Check sheet for the modelled part. Datum: model origin and axes. Units: mm. A direction names the side the tool comes from. Round coordinates to 2 decimals unless told otherwise and drop trailing zeros. Loops run counter-clockwise (first coordinate to the right, second up) from the corner with the lowest first, then second, coordinate; pieces in that order, holes last. Notation, with made-up numbers: (75, -37) - (86, -37) arc R21 cw to (86, -33) - close; hole circle Ø2 at (-14.75, 66). An arc over 180 degrees is marked (long way). Put each result on its own line as item: value.
```python
from build123d import *

# Parameters (mm, degrees)
SKETCH1_W           = 10
SKETCH1_H           = 32
BOSS_EXTRUDE1_DEPTH = 4
SKETCH2_R           = 2.5
CUT_EXTRUDE1_DEPTH  = 4
SKETCH3_W           = 10
SKETCH3_H           = 3
BOSS_EXTRUDE2_DEPTH = 28.76
SKETCH4_W           = 2.542985542
SKETCH4_H           = 9.222544282
BOSS_EXTRUDE3_DEPTH = 3
SKETCH5_R           = 2
CUT_EXTRUDE2_DEPTH  = 13


with BuildPart() as part:
    # Sketch1 → Boss-Extrude1 (new body)
    with BuildSketch(Plane(origin=(0, 0, 0), x_dir=(1, 0, 0), z_dir=(0, 1, 0))):
        with Locations((5, 16)):
            Rectangle(SKETCH1_W, SKETCH1_H)
    extrude(amount=BOSS_EXTRUDE1_DEPTH)

    # Sketch2 → Cut-Extrude1 (cut)
    with BuildSketch(Plane(origin=(0, 4, 0), x_dir=(1, 0, 0), z_dir=(0, 1, 0))):
        with Locations((5, 10)):
            Circle(SKETCH2_R)
    extrude(amount=-CUT_EXTRUDE1_DEPTH, mode=Mode.SUBTRACT)

    # Sketch3 → Boss-Extrude2 (add)
    with BuildSketch(Plane(origin=(0, 4, 0), x_dir=(1, 0, 0), z_dir=(0, 1, 0))):
        with Locations((5, 30.5)):
            Rectangle(SKETCH3_W, SKETCH3_H)
    extrude(amount=BOSS_EXTRUDE2_DEPTH)

    # Sketch4 → Boss-Extrude3 (add)
    with BuildSketch(Plane.XY.offset(-29)):
        Polygon((10, 37.329817811), (10, 46.552362093), (0, 46.552362093), (0, 29.76), (10, 29.76), align=None)
        with Locations((11.271492771, 41.941089952)):
            Rectangle(SKETCH4_W, SKETCH4_H)
    extrude(amount=BOSS_EXTRUDE3_DEPTH)

    # Sketch5 → Cut-Extrude2 (cut)
    with BuildSketch(Plane.XY.offset(-26)):
        with Locations((6.030433289, 41.199403662)):
            Circle(SKETCH5_R)
    extrude(amount=-CUT_EXTRUDE2_DEPTH, mode=Mode.SUBTRACT)


solid = part.part
```
Item 1: Section check B-B on z = -10. Enter the section's corners in (x, y).
Filled sheet:
outline: (0, 0) - (2.5, 0) - (2.5, 4) - (0, 4) - close; (7.5, 0) - (10, 0) - (10, 4) - (7.5, 4) - close
Item 2: Section check A-A on x = 3.5. Enter the section's corners in (y, z), then the cut area to 3 significant figures.
Filled sheet:
outline: (0, -32) - (32.76, -32) - (32.76, -29) - (46.55, -29) - (46.55, -26) - (29.76, -26) - (29.76, -29) - (4, -29) - (4, -12) - (0, -12) - close; (0, -8) - (4, -8) - (4, 0) - (0, 0) - close
area: 249 mm²
Item 3: Tool access check on faces 4 (the flat face through (5, 17, -29)), 5 (the flat face through (6, 38, -26)), 6 (the flat face through (5, 2, 0)), 7 (the flat face through (11, 37.33, -28)). Record the directions out of +Z, -Z, +X, -X, +Y, -Y that give a thin tool (end or side, any length) a straight path to the whole face; none if there is none.
Filled sheet:
face 4: +Z, +X, -X
face 5: +Z, +X, -X, +Y
face 6: +Z, +X, -X, +Y, -Y
face 7: +Z, -Z, +X, -Y
Item 4: Thickness scan on line 1 (Z direction, x = 5, y = 1.4); line 2 (Y direction, x = 1.5, z = -17.5); line 3 (Y direction, x = 3.5, z = -31). Record the ranges inside material, lowest first. Write a range as from..to.
Filled sheet:
line 1: -32..-12.5, -7.5..0
line 2: 0..4
line 3: 0..32.76
Item 5: Section check D-D on z = -28. Enter the section's corners in (x, y).
Filled sheet:
outline: (0, 0) - (10, 0) - (10, 4) - (0, 4) - close; (0, 29.76) - (10, 29.76) - (10, 37.33) - (12.54, 37.33) - (12.54, 46.55) - (0, 46.55) - close; hole circle Ø4 at (6.03, 41.2)
Item 6: Go/stop test with flat-tipped pins: pin 1 (3.5 mm diameter, centred on x = 3, z = -31, fed in from +Y); pin 2 (6 mm diameter, centred on x = 6.5, y = 39.5, fed in from -Z); pin 3 (4 mm diameter, centred on x = 2.5, z = -17.5, fed in from +Y); pin 4 (3.5 mm diameter, centred on x = 6.03, y = 41.2, fed in from +Z). Record where each tip stops, or that it passes through.
Filled sheet:
pin 1: y = 32.76
pin 2: z = -29
pin 3: y = 4
pin 4: through
Item 7: Section check C-C on x = 7. Enter the section's corners in (y, z), then the cut area to 3 significant figures.
Filled sheet:
outline: (0, -32) - (32.76, -32) - (32.76, -29) - (39.45, -29) - (39.45, -26) - (29.76, -26) - (29.76, -29) - (4, -29) - (4, -11.5) - (0, -11.5) - close; (0, -8.5) - (4, -8.5) - (4, 0) - (0, 0) - close; (42.95, -29) - (46.55, -29) - (46.55, -26) - (42.95, -26) - close
area: 242 mm²
Item 8: Release check for a two-part mould opening along Y. For faces 1 (the flat face through (5, 32.76, -31)), 2 (the flat face through (5, 29.76, -28)), 3 (the flat face through (8, 40, -29)) record: +Y half, -Y half, draft (parallel to the pull), parting line (faces both ways), or undercut.
Filled sheet:
face 1: +Y half
face 2: undercut
face 3: draft
